from build123d import *

# Parameters (mm, degrees)
BOSS_EXTRUDE1_DEPTH              = 38.1
F_13_64_0_20313_DIAMETER_HOLE1_D = 5.159375
F_1_4_0_25_DIAMETER_HOLE2_D      = 6.35
FILLET1_R                        = 9.525


with BuildPart() as part:
    # Sketch1 → Boss-Extrude1 (new body)
    with BuildSketch(Plane.XY):
        Polygon((0, 0), (0, 25.4), (3.175, 25.4), (3.175, 3.175), (38.1, 3.175), (38.1, 0), align=None)
    extrude(amount=BOSS_EXTRUDE1_DEPTH)

    # 13/64 (0.20313) Diameter Hole1 (through all)
    with Locations(Plane(origin=(0, 0, 0), x_dir=(-1, 0, 0), z_dir=(0, -1, 0))):
        with Locations((-25.4, -25.4), (-25.4, -12.065)):
            Hole(F_13_64_0_20313_DIAMETER_HOLE1_D / 2)

    # 1/4 (0.25) Diameter Hole2 (through all)
    with Locations(Plane.ZY):
        with Locations((19.05, 17.4625)):
            Hole(F_1_4_0_25_DIAMETER_HOLE2_D / 2)

    # Fillet1
    fillet1_edges = [part.edges().sort_by_distance(p)[0] for p in [
        (1.5875, 25.4, 38.1),
        (1.5875, 25.4, 0),
    ]]
    fillet(fillet1_edges, radius=FILLET1_R)


solid = part.part
Design review of the part built by this model. Coordinates are the model's own, in mm. A direction names the side the tool comes from. Round coordinates to 2 decimals unless told otherwise and drop trailing zeros. Write each loop counter-clockwise with the first axis right and the second up, starting at its lowest first coordinate (ties: lowest second). Pieces come first, ordered by that corner, then holes.
Item 1: Consider section A-A on z = 25.4. Give the boundary of the cut face in (x, y) (3 decimals), and give its area (3 significant figures).
Item 2: Consider section D-D on x = 33.5. Give the boundary of the cut face in (y, z) (3 decimals), and give its area (3 significant figures).
Item 3: Consider section C-C on z = 19.05. Give the boundary of the cut face in (x, y) (1 decimal), and give its area (3 significant figures).
Item 4: For faces 1 (the flat face through (3.175, 12, 19)), 2 (the cylindrical face through (1.61, 22.54, 35.38)), list the 3-axis set-ups (+Z, -Z, +X, -X, +Y, -Y) from which the entire face can be reached by the end or side of a thin tool; tool diameter is ignored.
Item 5: Consider section B-B on x = 24. Give the boundary of the cut face in (y, z) (3 decimals).
Item 6: Draft analysis for pull direction Z (two halves, no side actions). For faces 3 (the flat face through (0, 13, 19)), 4 (the cylindrical face through (22.823, 1.61, 25.287)), 5 (the cylindrical face through (1.61, 22.54, 2.72)), state which applies: released by +Z, released by -Z, zero draft, split by the parting line, or undercut.
Item 7: Wall thickness on L1, parallel to Z at x = 25.4, y = 0.6; L2, parallel to X at y = 2.5, z = 25.4; L3, parallel to Y at x = 2.25, z = 19.05: over which ranges is each line inside the solid? List them lowest first.
Item 8: For pin 1 Ø10 at (x, z) = (19.5, 24.5) entering from +Y (3 decimals); pin 2 Ø8 at (y, z) = (14, 33.5) entering from +X (3 decimals); pin 3 Ø4 at (x, z) = (25.4, 25.4) entering from +Y, all flat-tipped, find the tip position at first contact; note any pin that passes through.
Check values:
1. outline: (0, 0) - (22.82, 0) - (22.82, 3.175) - (3.175, 3.175) - (3.175, 25.4) - (0, 25.4) - close; (27.98, 0) - (38.1, 0) - (38.1, 3.175) - (27.98, 3.175) - close
1. area: 175 mm2
2. outline: (0, 0) - (3.175, 0) - (3.175, 38.1) - (0, 38.1) - close
2. area: 121 mm2
3. outline: (0, 0) - (38.1, 0) - (38.1, 3.2) - (3.2, 3.2) - (3.2, 14.3) - (0, 14.3) - close; (0, 20.6) - (3.2, 20.6) - (3.2, 25.4) - (0, 25.4) - close
3. area: 171 mm2
4. face 1: +Z, -Z, +X, +Y
4. face 2: +Z, +X, -X, +Y
5. outline: (0, 0) - (3.175, 0) - (3.175, 9.898) - (0, 9.898) - close; (0, 14.232) - (3.175, 14.232) - (3.175, 23.233) - (0, 23.233) - close; (0, 27.567) - (3.175, 27.567) - (3.175, 38.1) - (0, 38.1) - close
6. face 3: zero draft
6. face 4: undercut
6. face 5: released by -Z
7. L1: z = 0 to 9.49, 14.64 to 22.82, 27.98 to 38.1
7. L2: x = 0 to 22.82, 27.98 to 38.1
7. L3: y = 0 to 14.29, 20.64 to 25.4
8. pin 1: stops at y = 3.175
8. pin 2: stops at x = 3.175
8. pin 3: passes through
